Could you check a few things on this drawing? It's one solid part, dimensions in mm from its lowest x, y, z. Give positions to 0.01 mm unless a question says otherwise; leave off trailing zeros. Loops run counter-clockwise (first coordinate to the right, second up) from the corner with the lowest first, then second, coordinate; pieces in that order, holes last. Notation, with made-up numbers: (-14.75, 74.25) - (3.25, 74.25) arc R22 cw to (3.25, 104.25) - close; hole circle Ø10 at (-18.75, -29). An arc over 180 degrees is marked (long way). Use a Markdown table: item, result.
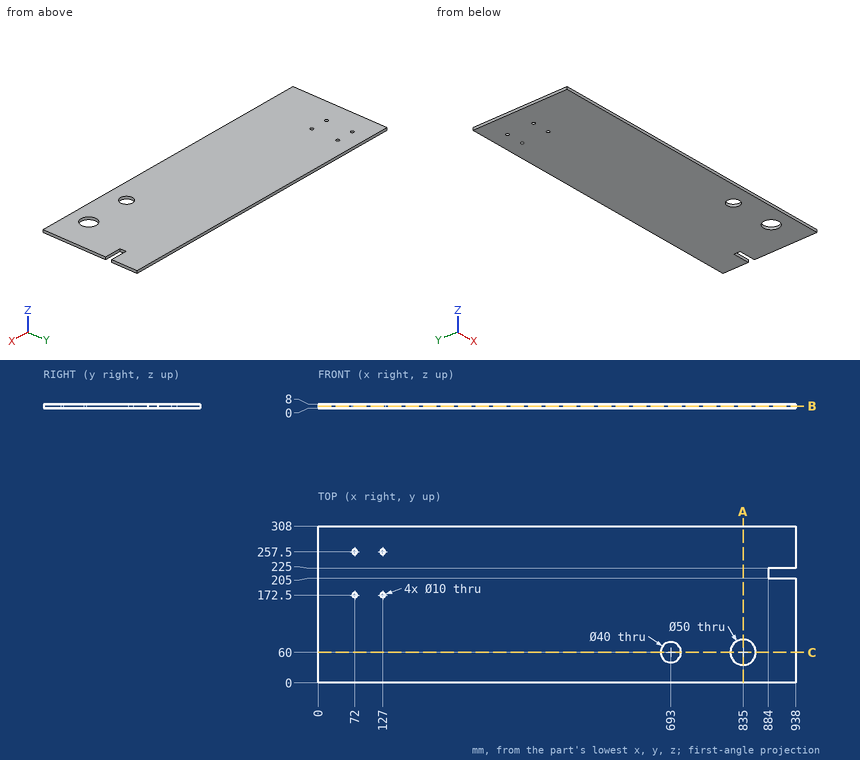
(1) Will this pin go through, and if not, where does the flat tip stop? pin 1 (9 mm diameter, centred on x = 127, y = 257.5, fed in from +Z).
A:
| item | result |
|---|---|
| pin 1 | through |
(2) Suppose I cut it at A-A on x = 835. Write out the boundary of the cut face in (y, z).
A:
| item | result |
|---|---|
| outline | (0, 0) - (35, 0) - (35, 8) - (0, 8) - close; (85, 0) - (308, 0) - (308, 8) - (85, 8) - close |
(3) Suppose I cut it at C-C on y = 60. Write out the boundary of the cut face in (x, z), plus the area to 3 significant figures.
A:
| item | result |
|---|---|
| outline | (0, 0) - (673, 0) - (673, 8) - (0, 8) - close; (713, 0) - (810, 0) - (810, 8) - (713, 8) - close; (860, 0) - (938, 0) - (938, 8) - (860, 8) - close |
| area | 6,780 mm2 |
(4) Suppose I cut it at B-B on z = 3.75. Write out the boundary of the cut face in (x, y), plus the area to 3 significant figures.
A:
| item | result |
|---|---|
| outline | (0, 0) - (938, 0) - (938, 205) - (884, 205) - (884, 225) - (938, 225) - (938, 308) - (0, 308) - close; hole circle Ø10 at (72, 172.5); hole circle Ø10 at (72, 257.5); hole circle Ø10 at (127, 172.5); hole circle Ø10 at (127, 257.5); hole circle Ø40 at (693, 60); hole circle Ø50 at (835, 60) |
| area | 284,000 mm2 |
(5) If I drill on line 1 (Y direction, x = 127, z = 5); line 2 (X direction, y = 59.5, z = 1) (3 decimals); line 3 (Y direction, x = 699, z = 1.5), over which ranges is the centre line in solid material (lowest first)?
A:
| item | result |
|---|---|
| line 1 | 0 to 167.5, 177.5 to 252.5, 262.5 to 308 |
| line 2 | 0 to 673.006, 712.994 to 810.005, 859.995 to 938 |
| line 3 | 0 to 40.92, 79.08 to 308 |
